Autodesk Inventor part; units mm, degrees
ref_plane "YZ Plane" through (0, 0, 0) normal (1, 0, 0) x (0, 1, 0)
ref_plane "XZ Plane" through (0, 0, 0) normal (0, 1, 0) x (-1, 0, 0)
ref_plane "XY Plane" through (0, 0, 0) normal (0, 0, 1) x (1, 0, 0)
sketch "Sketch1" plane through (0, 0, 0) normal (0, 1, 0) x (-1, 0, 0)
  circle A0 centre (0, 0) radius 23
  circle A1 centre (0, 0) radius 20
  dimension "d0" = 3
  dimension "d1" = 40
extrude "Extrusion1" add sketch "Sketch1" along normal blind 150
sketch "Sketch2" plane through (0, 0, 0) normal (0, 0, 1) x (1, 0, 0)
  line L0 (-23, 135) -> (0, 135)
  line L1 (0, 135) -> (0, 60)
  line L2 (0, 60) -> (-23, 60)
  line L3 (-23, 60) -> (-23, 135)
  line L4 (23, 150) -> (-23, 150)
  line L5 (-23, 0) -> (23, 0)
  point P0 (0, 0)
  dimension "d4" = 75
  dimension "d19" = 15
extrude "Extrusion2" cut sketch "Sketch2" along normal mid plane 25
fillet "Fillet1" radius 5 4 edges at (-17.4596, 135, -12.5) (-17.4596, 135, 12.5) (-17.4596, 60, 12.5) (-17.4596, 60, -12.5)
sketch "Sketch3" plane through (0, 0, 0) normal (1, 0, 0) x (0, 1, 0)
  line L0 (-20, 0) -> (120, 0)
  line L1 (135, -7.5) -> (135, 7.5)
  line L2 (150, 20) -> (150, -20)
  point P0 (0, 0)
  point P1 (130, 0)
  point P2 (100, 0)
  dimension "d9" = 30
  dimension "d18" = 20
hole "Hole1" at (0, 130, 0) at (0, 100, 0) direction (1, 0, 0) diameter 4.5 end through all
properties part number "Pancake_PVC Pipe Long" material "PVC-Piping"
For this review, take the finished solid that the model builds, in its own axes (mm). A direction names the side the tool comes from. Give positions to 0.01 mm unless a question says otherwise; leave off trailing zeros. Write each loop counter-clockwise with the first axis right and the second up, starting at its lowest first coordinate (ties: lowest second). Pieces come first, ordered by that corner, then holes. Notation, with made-up numbers: (-0.5, 47) -> (35.5, 47) arc R14 ccw to (35.5, 66) -> close; hole circle Ø11 at (32.25, -27.75). An arc over 180 degrees is marked (long way). Use CSV: the item, a comma, the result in double quotes.
Q1. Take a section at A-A, the plane z = 0. Write out the cut boundary in (x, y).
Conclusion:
outline,"(-23, 0) -> (-20, 0) -> (-20, 60) -> (-23, 60) -> close; (-23, 135) -> (-20, 135) -> (-20, 150) -> (-23, 150) -> close; (20, 0) -> (23, 0) -> (23, 97.75) -> (20, 97.75) -> close; (20, 102.25) -> (23, 102.25) -> (23, 127.75) -> (20, 127.75) -> close; (20, 132.25) -> (23, 132.25) -> (23, 150) -> (20, 150) -> close"
Q2. Take a section at C-C, the plane z = -17.5. Write out the cut boundary in (x, y).
Conclusion:
outline,"(-14.92, 0) -> (-9.68, 0) -> (-9.68, 150) -> (-14.92, 150) -> close; (9.68, 0) -> (14.92, 0) -> (14.92, 150) -> (9.68, 150) -> close"
Q3. For P1, Ø10, axis at x = -3, y = 32, coming from the +Z side; P2, Ø10, axis at x = 18, y = 105.5, coming from the +Z side; P3, Ø2, axis at y = 126, z = -17.5, coming from the +X side, all flat-tipped, find the tip position at first contact; note any pin that passes through.
Conclusion:
P1,"z = 23"
P2,"z = 18.97"
P3,"x = 16.02"
Q4. Mouldability with a two-part tool opening along Y and no side actions: class faces 3 (the face through (-21, 135, 0)), 4 (the face through (7, 0, 19)), 5 (the face through (7, 150, 19)) as pulls with the +Y half, pulls with the -Y half, needs draft (parallel to the pull), parting line crosses it, or undercut.
Conclusion:
face 3,"undercut"
face 4,"pulls with the -Y half"
face 5,"pulls with the +Y half"
Q5. Take a section at B-B, the plane x = 0. Write out the cut boundary in (y, z).
Conclusion:
outline,"(0, -23) -> (150, -23) -> (150, -20) -> (0, -20) -> close; (0, 20) -> (150, 20) -> (150, 23) -> (0, 23) -> close"
Q6. Tool access review of faces 1 (the face through (-18.72, 61.43, 11)), 2 (the face through (21.458, 132.196, -0.488)): name each direction out of +Z, -Z, +X, -X, +Y, -Y from which nothing blocks a thin tool from reaching the whole face with its end or side.
Conclusion:
face 1,"-X"
face 2,"+X, -X"
Q7. Take a section at D-D, the plane y = 53. Write out the cut boundary in (x, z), then the cut area to 3 significant figures.
Conclusion:
outline,"circle Ø46 at (0, 0); hole circle Ø40 at (0, 0)"
area,"405 mm2"
Q8. To check wall thickness, follow probe 1 along X at (y, z) = (40, 0); probe 2 along Z at (x, y) = (-13, 123); probe 3 along X at (y, z) = (105, 0). State the ranges of each line that lie inside material, in increasing order. Write a range as [from, to].
Conclusion:
probe 1,"[-23, -20], [20, 23]"
probe 2,"[-18.97, -15.2], [15.2, 18.97]"
probe 3,"[20, 23]"
